```python
from build123d import *

# Parameters (mm, degrees)
CROQUIS1_W              = 214
CROQUIS1_H              = 73.64
SALIENTE_EXTRUIR1_DEPTH = 3
CROQUIS3_W              = 3
CROQUIS3_H              = 6
SALIENTE_EXTRUIR2_DEPTH = 3
CROQUIS2_R              = 4
CORTAR_EXTRUIR1_DEPTH   = 4
CROQUIS5_R              = 1.55
CORTAR_EXTRUIR3_DEPTH   = 4
CROQUIS6_W              = 72.45
CROQUIS6_H              = 27.8
CORTAR_EXTRUIR4_DEPTH   = 4


with BuildPart() as part:
    # Croquis1 → Saliente-Extruir1 (new body)
    with BuildSketch(Plane(origin=(0, 0, 0), x_dir=(1, 0, 0), z_dir=(0, 1, 0))):
        Rectangle(CROQUIS1_W, CROQUIS1_H)
    extrude(amount=SALIENTE_EXTRUIR1_DEPTH)

    # Croquis3 → Saliente-Extruir2 (add, through all)
    with BuildSketch(Plane(origin=(0, 3, 0), x_dir=(1, 0, 0), z_dir=(0, 1, 0))):
        with Locations((-108.5, 23.82)):
            Rectangle(CROQUIS3_W, CROQUIS3_H)
        with Locations((-108.5, -23.82)):
            Rectangle(CROQUIS3_W, CROQUIS3_H)
        with Locations((108.5, 23.82)):
            Rectangle(CROQUIS3_W, CROQUIS3_H)
        with Locations((108.5, -23.82)):
            Rectangle(CROQUIS3_W, CROQUIS3_H)
    extrude(amount=-SALIENTE_EXTRUIR2_DEPTH)

    # Croquis2 → Cortar-Extruir1 (cut, through all)
    with BuildSketch(Plane(origin=(0, 3, 0), x_dir=(1, 0, 0), z_dir=(0, 1, 0))):
        with Locations((0, -22.18)):
            Circle(CROQUIS2_R)
    extrude(amount=-CORTAR_EXTRUIR1_DEPTH, mode=Mode.SUBTRACT)

    # Croquis5 → Cortar-Extruir3 (cut, through all)
    with BuildSketch(Plane(origin=(0, 3, 0), x_dir=(1, 0, 0), z_dir=(0, 1, 0))):
        with Locations((-60.15, 23.604994207)):
            Circle(CROQUIS5_R)
        with Locations((37.85, 23.604994207)):
            Circle(CROQUIS5_R)
        with Locations((37.85, -7.595005793)):
            Circle(CROQUIS5_R)
        with Locations((-60.15, -7.595005793)):
            Circle(CROQUIS5_R)
    extrude(amount=-CORTAR_EXTRUIR3_DEPTH, mode=Mode.SUBTRACT)

    # Croquis6 → Cortar-Extruir4 (cut, through all)
    with BuildSketch(Plane(origin=(0, 3, 0), x_dir=(1, 0, 0), z_dir=(0, 1, 0))):
        with Locations((0.575, 7.604994207)):
            Rectangle(CROQUIS6_W, CROQUIS6_H)
    extrude(amount=-CORTAR_EXTRUIR4_DEPTH, mode=Mode.SUBTRACT)


solid = part.part
```
Can you work these out from the model? Positions are in its coordinate system, mm. Give positions to 0.01 mm unless a question says otherwise; leave off trailing zeros. Write each loop counter-clockwise with the first axis right and the second up, starting at its lowest first coordinate (ties: lowest second). Pieces come first, ordered by that corner, then holes. Notation, with made-up numbers: (89.5, 47) -> (119.5, 47) arc R25 ccw to (119.5, 81) -> close; hole circle Ø8 at (82, 45.5). An arc over 180 degrees is marked (long way). One line per item, written item: value.
Q1. We'd pull the mould along Z, two halves only. Please class faces 1 (the face through (-2, 3, 8)), 2 (the face through (-0.867, 1.521, 26.085)): +Z half, -Z half, draft (parallel to the pull), parting line (faces both ways), or undercut.
Results found:
face 1: draft
face 2: undercut
Q2. Please list where these lines run through material, in increasing order: line 1 (Z direction, x = 37.85, y = 1.1) (3 decimals); line 2 (X direction, y = 1.15, z = -5.5); line 3 (Z direction, x = 0, y = 1.75) (3 decimals). Write a range as [from, to].
Results found:
line 1: z = [-36.82, -25.155], [-22.055, 6.045], [9.145, 36.82]
line 2: x = [-107, -35.65], [36.8, 107]
line 3: z = [-36.82, -21.505], [6.295, 18.18], [26.18, 36.82]
Q3. Imagine slicing it at A-A on z = -4. Please give me the cut outline in (x, y), and give its area (3 significant figures).
Results found:
outline: (-107, 0) -> (-35.65, 0) -> (-35.65, 3) -> (-107, 3) -> close; (36.8, 0) -> (107, 0) -> (107, 3) -> (36.8, 3) -> close
area: 425 mm^2
Q4. Imagine slicing it at C-C on y = 0.65. Give the number of separate pieces and of enclosed holes in the cut face, and give its area (3 significant figures).
Results found:
separate pieces: 1
enclosed holes: 6
area: 13,700 mm^2
Q5. Imagine slicing it at B-B on x = 0. Please give me the cut outline in (y, z) (3 decimals), and give its area (3 significant figures).
Results found:
outline: (0, -36.82) -> (3, -36.82) -> (3, -21.505) -> (0, -21.505) -> close; (0, 6.295) -> (3, 6.295) -> (3, 18.18) -> (0, 18.18) -> close; (0, 26.18) -> (3, 26.18) -> (3, 36.82) -> (0, 36.82) -> close
area: 114 mm^2
Q6. For P1, Ø1.5, axis at y = 1.5, z = 33, coming from the +X side; P2, Ø1.5, axis at x = -108.5, y = 1, coming from the -Z side; P3, Ø1.5, axis at y = 2, z = -32, coming from the -X side, each with a flat end and sliding along its axis, tell me the tip position at first contact or that it passes through.
Results found:
P1: stops at x = 107
P2: stops at z = -26.82
P3: stops at x = -107
